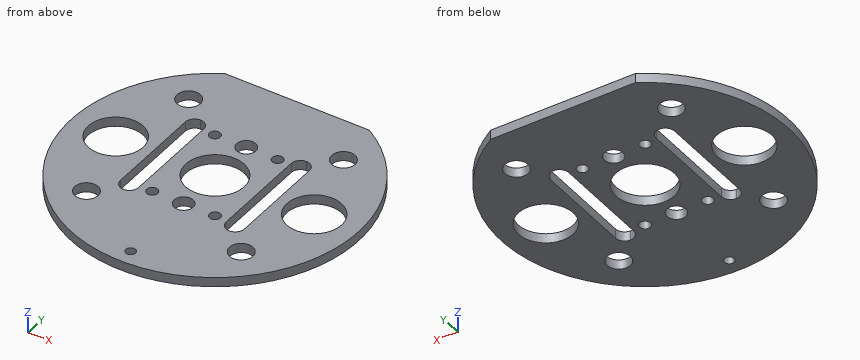
from build123d import *

# Parameters (mm, degrees)
SKETCH_1_R               = 50
EXTRUDE_1_DEPTH          = 3.302
SKETCH_2_R               = 4.064
CUT_EXTRUDE_1_DEPTH      = 71.787733429
SKETCH_3_W               = 50.417758776
SKETCH_3_H               = 15.226983209
CUT_EXTRUDE_2_DEPTH      = 71.787733429
SKETCH_4_R               = 10.16
CUT_EXTRUDE_3_DEPTH      = 71.787733429
SKETCH_8_R               = 9.525
SKETCH_8_W               = 6.35
SKETCH_8_H               = 40.64
CUT_EXTRUDE_4_DEPTH      = 71.787733429
SKETCH_9_R               = 1.9
SKETCH_9_R_2             = 3.302
CUT_EXTRUDE_5_DEPTH      = 71.787733429
FILLET1_R                = 3.175
M3_CLEARANCE_HOLE1_D     = 3.4
M3_CLEARANCE_HOLE1_DEPTH = 25.4
M3_CLEARANCE_HOLE1_TIP   = 1.021463052


with BuildPart() as part:
    # 草图1 → 凸台-拉伸1 (new body)
    with BuildSketch(Plane.XY):
        with Locations(Location((0, 0, 0), (0, 0, 180))):
            Circle(SKETCH_1_R)
    extrude(amount=EXTRUDE_1_DEPTH)

    # 草图2 → 切除-拉伸1 (cut, through all)
    with BuildSketch(Plane.XY.offset(3.302)):
        with Locations((-26.940768363, 26.940768363)):
            Circle(SKETCH_2_R)
        with Locations((-26.940768363, -26.940768363)):
            Circle(SKETCH_2_R)
        with Locations((26.940768363, -26.940768363)):
            Circle(SKETCH_2_R)
        with Locations((26.940768363, 26.940768363)):
            Circle(SKETCH_2_R)
    extrude(amount=-CUT_EXTRUDE_1_DEPTH, mode=Mode.SUBTRACT)

    # 草图3 → 切除-拉伸2 (cut, through all)
    with BuildSketch(Plane.XY.offset(3.302)):
        with Locations((0, 50.793491605)):
            Rectangle(SKETCH_3_W, SKETCH_3_H)
    extrude(amount=-CUT_EXTRUDE_2_DEPTH, mode=Mode.SUBTRACT)

    # 草图4 → 切除-拉伸3 (cut, through all)
    with BuildSketch(Plane.XY.offset(3.302)):
        Circle(SKETCH_4_R)
    extrude(amount=-CUT_EXTRUDE_3_DEPTH, mode=Mode.SUBTRACT)

    # 草图8 → 切除-拉伸4 (cut, through all)
    with BuildSketch(Plane.XY.offset(3.302)):
        with Locations((34.544, 0)):
            Circle(SKETCH_8_R)
        with Locations((-34.544, 0)):
            Circle(SKETCH_8_R)
        with Locations((18.415, 0)):
            Rectangle(SKETCH_8_W, SKETCH_8_H)
        with Locations((-18.415, 0)):
            Rectangle(SKETCH_8_W, SKETCH_8_H)
    extrude(amount=-CUT_EXTRUDE_4_DEPTH, mode=Mode.SUBTRACT)

    # 草图9 → 切除-拉伸5 (cut, through all)
    with BuildSketch(Plane.XY.offset(3.302)):
        with Locations((-10.922, 16.51)):
            Circle(SKETCH_9_R)
        with Locations((10.922, 16.51)):
            Circle(SKETCH_9_R)
        with Locations((-10.922, -16.51)):
            Circle(SKETCH_9_R)
        with Locations((10.922, -16.51)):
            Circle(SKETCH_9_R)
        with Locations((0, 16.51)):
            Circle(SKETCH_9_R_2)
        with Locations((0, -16.51)):
            Circle(SKETCH_9_R_2)
    extrude(amount=-CUT_EXTRUDE_5_DEPTH, mode=Mode.SUBTRACT)

    # Fillet1
    fillet1_edges = [part.edges().sort_by_distance(p)[0] for p in [
        (15.24, 20.32, 1.651),
        (21.59, 20.32, 1.651),
        (21.59, -20.32, 1.651),
        (15.24, -20.32, 1.651),
        (-15.24, -20.32, 1.651),
        (-21.59, -20.32, 1.651),
        (-15.24, 20.32, 1.651),
        (-21.59, 20.32, 1.651),
    ]]
    fillet(fillet1_edges, radius=FILLET1_R - 0.0001)  # a hair under: the kernel refuses the full size

    # M3 Clearance Hole1
    with Locations(Plane.XY.offset(3.302)):
        with Locations((0, -44.45)):
            Hole(M3_CLEARANCE_HOLE1_D / 2, depth=M3_CLEARANCE_HOLE1_DEPTH)
            with Locations((0, 0, -(M3_CLEARANCE_HOLE1_DEPTH + M3_CLEARANCE_HOLE1_TIP / 2))):  # 118° drill point
                Cone(0, M3_CLEARANCE_HOLE1_D / 2, M3_CLEARANCE_HOLE1_TIP, mode=Mode.SUBTRACT)


solid = part.part
Can you work these out from the model? Positions are in its coordinate system, mm. Give positions to 0.01 mm unless a question says otherwise; leave off trailing zeros. Write each loop counter-clockwise with the first axis right and the second up, starting at its lowest first coordinate (ties: lowest second). Pieces come first, ordered by that corner, then holes. Notation, with made-up numbers: (88, 41) -> (104, 41) arc R21 ccw to (104, 64) -> close; hole circle Ø11 at (7.5, 86). An arc over 180 degrees is marked (long way). Answer as a JSON object with one key per item and string values. Group by question number.
Item 1: Suppose I cut it at C-C (y = -44.45). Please give me the cut outline in (x, z), plus the area to 3 significant figures.
Item 2: Suppose I cut it at B-B (y = 0). Please give me the cut outline in (x, z).
Item 3: Please list where these lines run through material, in increasing order: line 1 (Y direction, x = 0, z = 2.15); line 2 (X direction, y = 5.5, z = 1.5); line 3 (X direction, y = 4, z = 1.2). Write a range as [from, to].
Item 4: Suppose I cut it at D-D (x = 41). Please give me the cut outline in (y, z), plus the area to 3 significant figures.
Item 5: I'm going to push flat-ended pins straight in: P1, Ø1, axis at y = 2.5, z = 2, coming from the +X side; P2, Ø1, axis at y = 29.5, z = 2.5, coming from the -X side. Where does each tip first touch, or does it pass through?
Item 6: Suppose I cut it at A-A (x = 0). Please give me the cut outline in (y, z), plus the area to 3 significant figures.
Findings:
{
 "1": {"outline": "(-22.9, 0) -> (-1.7, 0) -> (-1.7, 3.3) -> (-22.9, 3.3) -> close; (1.7, 0) -> (22.9, 0) -> (22.9, 3.3) -> (1.7, 3.3) -> close", "area": "140 mm²"},
 "2": {"outline": "(-50, 0) -> (-44.07, 0) -> (-44.07, 3.3) -> (-50, 3.3) -> close; (-25.02, 0) -> (-21.59, 0) -> (-21.59, 3.3) -> (-25.02, 3.3) -> close; (-15.24, 0) -> (-10.16, 0) -> (-10.16, 3.3) -> (-15.24, 3.3) -> close; (10.16, 0) -> (15.24, 0) -> (15.24, 3.3) -> (10.16, 3.3) -> close; (21.59, 0) -> (25.02, 0) -> (25.02, 3.3) -> (21.59, 3.3) -> close; (44.07, 0) -> (50, 0) -> (50, 3.3) -> (44.07, 3.3) -> close"},
 "3": {"line 1": "y = [-50, -46.15], [-42.75, -19.81], [-13.21, -10.16], [10.16, 13.21], [19.81, 43.18]", "line 2": "x = [-49.7, -42.32], [-26.77, -21.59], [-15.24, -8.54], [8.54, 15.24], [21.59, 26.77], [42.32, 49.7]", "line 3": "x = [-49.84, -43.19], [-25.9, -21.59], [-15.24, -9.34], [9.34, 15.24], [21.59, 25.9], [43.19, 49.84]"},
 "4": {"outline": "(-28.62, 0) -> (-7, 0) -> (-7, 3.3) -> (-28.62, 3.3) -> close; (7, 0) -> (28.62, 0) -> (28.62, 3.3) -> (7, 3.3) -> close", "area": "143 mm²"},
 "5": {"P1": "stops at x = 49.96", "P2": "stops at x = -40.73"},
 "6": {"outline": "(-50, 0) -> (-46.15, 0) -> (-46.15, 3.3) -> (-50, 3.3) -> close; (-42.75, 0) -> (-19.81, 0) -> (-19.81, 3.3) -> (-42.75, 3.3) -> close; (-13.21, 0) -> (-10.16, 0) -> (-10.16, 3.3) -> (-13.21, 3.3) -> close; (10.16, 0) -> (13.21, 0) -> (13.21, 3.3) -> (10.16, 3.3) -> close; (19.81, 0) -> (43.18, 0) -> (43.18, 3.3) -> (19.81, 3.3) -> close", "area": "186 mm²"}
}
